Read the model definition and answer for the solid it produces. Units are mm, in the model's axes. Round coordinates to 2 decimals unless told otherwise and drop trailing zeros. Answer as CSV lines item,"result". Start each with the question number.
1) Consider line 1 along X through (y, z) = (-41.5, 186.5); line 2 along X through (y, z) = (43, 67.5); line 3 along Z through (x, y) = (-29, -45.5). Determine where each line is inside the solid, lowest interval first.
2) This flat-tipped pin is pushed along its axis until it touches: pin 1 (6 mm diameter, centred on x = -20, y = -27, fed in from -Z). Where does it stop, or does it pass through?
3) For a pull along X with two mould halves and no side action, classify faces 1 (the flat face through (1, -46, 196)), 2 (the cylindrical face through (47.15, -46.99, 98.71)), 3 (the flat face through (-50, 1, 99)) as +X half, -X half, draft (parallel to the pull), parting line (faces both ways), or undercut.
Autodesk Inventor part; units mm, degrees
ref_plane "YZ Plane" through (0, 0, 0) normal (1, 0, 0) x (0, 1, 0)
ref_plane "XZ Plane" through (0, 0, 0) normal (0, 1, 0) x (-1, 0, 0)
ref_plane "XY Plane" through (0, 0, 0) normal (0, 0, 1) x (1, 0, 0)
sketch "Skizze1" plane through (0, 0, 0) normal (0, 0, 1) x (1, 0, 0)
  line L0 (-40, -50) -> (40, -50)
  line L1 (50, -40) -> (50, 40)
  line L2 (40, 50) -> (-40, 50)
  line L3 (-50, 40) -> (-50, -40)
  line L4 (-50, -50) -> (50, 50) construction
  line L5 (50, -50) -> (-50, 50) construction
  arc A0 (-40, 50) -> (-50, 40) centre (-40, 40) ccw
  arc A1 (50, 40) -> (40, 50) centre (40, 40) ccw
  arc A2 (40, -50) -> (50, -40) centre (40, -40) ccw
  arc A3 (-50, -40) -> (-40, -50) centre (-40, -40) ccw
  point P0 (0, 0)
  dimension "d0" = 100
  dimension "d1" = 100
  dimension "d2" = 10
extrude "Extrusion1" add sketch "Skizze1" along normal blind 200
chamfer "Fase1" distance 8 angle 45 16 edges at (50, 0, 200) (47.0711, 47.0711, 200) (0, 50, 200) (-47.0711, 47.0711, 200) (-50, 0, 200) (-47.0711, -47.0711, 200) (0, -50, 200) (47.0711, -47.0711, 200) (50, 0, 0) (47.0711, 47.0711, 0) (0, 50, 0) (-47.0711, 47.0711, 0) (-50, 0, 0) (-47.0711, -47.0711, 0) (0, -50, 0) (47.0711, -47.0711, 0)
properties part number "Motor"
Check values:
1,line 1,"x = -49.89 to 49.89"
1,line 2,"x = -49.54 to 49.54"
1,line 3,"z = 3.5 to 196.5"
2,pin 1,"stops at z = 0"
3,face 1,"draft"
3,face 2,"+X half"
3,face 3,"-X half"
